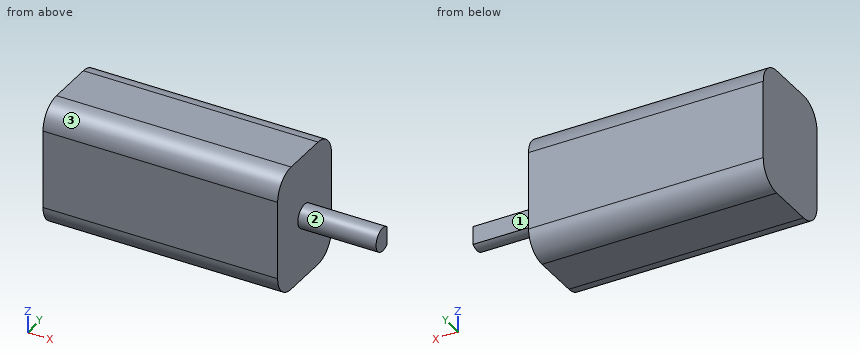
```python
from build123d import *

# Parameters (mm, degrees)
SKETCH1_W           = 30
SKETCH1_H           = 16
BOSS_EXTRUDE1_DEPTH = 12
FILLET2_R           = 3
BOSS_EXTRUDE3_DEPTH = 10


with BuildPart() as part:
    # Sketch1 → Boss-Extrude1 (new body)
    with BuildSketch(Plane(origin=(0, 0, 0), x_dir=(1, 0, 0), z_dir=(0, 1, 0))):
        Rectangle(SKETCH1_W, SKETCH1_H)
    extrude(amount=BOSS_EXTRUDE1_DEPTH)

    # Fillet2
    fillet2_edges = [part.edges().sort_by_distance(p)[0] for p in [
        (0, 12, 8),
        (0, 0, 8),
        (0, 0, -8),
        (0, 12, -8),
    ]]
    fillet(fillet2_edges, radius=FILLET2_R)

    # Sketch3 → Boss-Extrude3 (add)
    with BuildSketch(Plane(origin=(15, 0, 0), x_dir=(0, 0, -1), z_dir=(1, 0, 0))):
        with BuildLine():
            Line((-1.166565174, 6.942934619), (1.166565174, 6.942934619))
            ThreePointArc((1.166565174, 6.942934619), (0, 4.5), (-1.166565174, 6.942934619))
        make_face()
    extrude(amount=BOSS_EXTRUDE3_DEPTH)


solid = part.part
```
Read the model definition and answer for the solid it produces. Units are mm, in the model's axes. Face numbers are marked on the shaded views. A direction names the side the tool comes from. Round coordinates to 2 decimals unless told otherwise and drop trailing zeros. Write each loop counter-clockwise with the first axis right and the second up, starting at its lowest first coordinate (ties: lowest second). Pieces come first, ordered by that corner, then holes. Notation, with made-up numbers: (58.5, 22.25) - (96.5, 22.25) arc R11 ccw to (96.5, 32.25) - close; hole circle Ø8 at (51.25, 61.25). An arc over 180 degrees is marked (long way). One line per item, written item: value.
Q1. Which of the six approach directions +Z, -Z, +X, -X, +Y, -Y give full straight-line access (tool end or side, diameter ignored) to the marked faces 1, 2 and 3?
The answers:
face 1: +Z, -Z, +X, +Y
face 2: +X
face 3: +Z, +X, -X, -Y
Q2. Straight lines are drawn through the part: line 1 (X direction, y = 11, z = 2); line 2 (Y direction, x = 2, z = -6); line 3 (Z direction, x = 21.5, y = 4.75). For each, find the intervals that lie inside material, in ascending order. Write a range as from..to.
The answers:
line 1: x = -15..15
line 2: y = 0.17..11.83
line 3: z = -0.83..0.83
Q3. Each of these flat-tipped pins is pushed along its axis until it touches: P1, Ø1, axis at y = 3.5, z = -2.5, coming from the +X side; P2, Ø0.7, axis at x = 22, z = 0.5, coming from the +Y side. Where does it stop, or does it pass through?
The answers:
P1: stops at x = 15
P2: stops at y = 6.94
Q4. Find section A-A (y = 6). Determine the outline of the cut face in (x, z).
The answers:
outline: (-15, -8) - (15, -8) - (15, -1.5) - (25, -1.5) - (25, 1.5) - (15, 1.5) - (15, 8) - (-15, 8) - close
Q5. Find section C-C (z = 4.25). Determine the outline of the cut face in (x, y).
The answers:
outline: (-15, 0) - (15, 0) - (15, 12) - (-15, 12) - close
Q6. Find section D-D (x = 21). Determine the outline of the cut face in (y, z).
The answers:
outline: (6.94, -1.17) - (6.94, 1.17) arc R1.5 ccw (long way) to start
Q7. Find section B-B (x = -10). Determine the outline of the cut face in (y, z).
The answers:
outline: (0, -5) arc R3 ccw to (3, -8) - (9, -8) arc R3 ccw to (12, -5) - (12, 5) arc R3 ccw to (9, 8) - (3, 8) arc R3 ccw to (0, 5) - close
